from build123d import *

# Parameters (mm, degrees)
BOX006_W               = 2
BOX006_H               = 10
BOX006_DEPTH           = 30
BOX005_W               = 2
BOX005_H               = 10
BOX005_DEPTH           = 30
CYLINDER001_R          = 7.7
CYLINDER001_DEPTH      = 25
CYLINDER_R             = 7.7
CYLINDER_DEPTH         = 25
BOX004_W               = 32
BOX004_H               = 10
BOX004_DEPTH           = 15
BOX004_PLACEMENT_ANGLE = -37
BOX_W                  = 60
BOX_H                  = 10
BOX_DEPTH              = 15
CYLINDER002_R          = 11
CYLINDER002_DEPTH      = 25
CYLINDER003_R          = 11
CYLINDER003_DEPTH      = 25
BOX003_W               = 34
BOX003_H               = 10
BOX003_DEPTH           = 15
BOX003_PLACEMENT_ANGLE = 37
BOX002_W               = 34
BOX002_H               = 10
BOX002_DEPTH           = 15
BOX002_PLACEMENT_ANGLE = 37
CYLINDER005_R          = 7.2
CYLINDER005_DEPTH      = 40
CYLINDER004_R          = 7.2
CYLINDER004_DEPTH      = 40
BOX001_W               = 60
BOX001_H               = 10
BOX001_DEPTH           = 15
CHAMFER_SIZE           = 3


with BuildPart() as cube006:
    # Box006 → Box006 (new body)
    with BuildSketch(Plane(origin=(59, -15, 0), x_dir=(1, 0, 0), z_dir=(0, 0, 1))):
        with Locations((1, 5)):
            Rectangle(BOX006_W, BOX006_H)
    extrude(amount=BOX006_DEPTH)


with BuildPart() as cube005:
    # Box005 → Box005 (new body)
    with BuildSketch(Plane(origin=(-1, -15, 0), x_dir=(1, 0, 0), z_dir=(0, 0, 1))):
        with Locations((1, 5)):
            Rectangle(BOX005_W, BOX005_H)
    extrude(amount=BOX005_DEPTH)


with BuildPart() as cylinder001:
    # Cylinder001 → Cylinder001 (new body)
    with BuildSketch(Plane(origin=(60, 0, 0), x_dir=(1, 0, 0), z_dir=(0, 0, 1))):
        Circle(CYLINDER001_R)
    extrude(amount=CYLINDER001_DEPTH)


with BuildPart() as cylinder:
    # Cylinder → Cylinder (new body)
    with BuildSketch(Plane.XY):
        Circle(CYLINDER_R)
    extrude(amount=CYLINDER_DEPTH)


with BuildPart() as cube004:
    # Box004 → Box004 (new body)
    with BuildSketch(Plane.XY):
        with Locations((16, 5)):
            Rectangle(BOX004_W, BOX004_H)
    extrude(amount=BOX004_DEPTH)


with BuildPart() as cube004_1:
    # Box004 placement: moved
    add(cube004.part.moved(Location((23, 20, 0))).rotate(Axis((23, 20, 0), (0, 0, 1)), BOX004_PLACEMENT_ANGLE))


with BuildPart() as cube:
    # Box → Box (new body)
    with BuildSketch(Plane.XY):
        with Locations((30, 5)):
            Rectangle(BOX_W, BOX_H)
    extrude(amount=BOX_DEPTH)


with BuildPart() as cylinder002:
    # Cylinder002 → Cylinder002 (new body)
    with BuildSketch(Plane.XY):
        Circle(CYLINDER002_R)
    extrude(amount=CYLINDER002_DEPTH)


with BuildPart() as fusion003:
    # Cylinder003 → Cylinder003 (new body)
    with BuildSketch(Plane(origin=(60, 0, 0), x_dir=(1, 0, 0), z_dir=(0, 0, 1))):
        Circle(CYLINDER003_R)
    extrude(amount=CYLINDER003_DEPTH)

    # Fusion: union Cube, Cylinder002
    add(cube.part)
    add(cylinder002.part)

    # Fusion003: union Cube004
    add(cube004_1.part)


with BuildPart() as fusion004:
    # Box003 → Box003 (new body)
    with BuildSketch(Plane.XY):
        with Locations((17, 5)):
            Rectangle(BOX003_W, BOX003_H)
    extrude(amount=BOX003_DEPTH)


with BuildPart() as fusion004_1:
    # Box003 placement: moved
    add(fusion004.part.moved(Location((60, 0, 0))).rotate(Axis((60, 0, 0), (0, 0, 1)), BOX003_PLACEMENT_ANGLE))

    # Fusion004: union Fusion003
    add(fusion003.part)


with BuildPart() as cut003:
    # Box002 → Box002 (new body)
    with BuildSketch(Plane.XY):
        with Locations((17, 5)):
            Rectangle(BOX002_W, BOX002_H)
    extrude(amount=BOX002_DEPTH)


with BuildPart() as cut003_1:
    # Box002 placement: moved
    add(cut003.part.rotate(Axis((0, 0, 0), (0, 0, 1)), BOX002_PLACEMENT_ANGLE))

    # Fusion005: union Fusion004
    add(fusion004_1.part)

    # Cut: cut Cylinder
    add(cylinder.part, mode=Mode.SUBTRACT)

    # Cut001: cut Cylinder001
    add(cylinder001.part, mode=Mode.SUBTRACT)

    # Cut002: cut Cube005
    add(cube005.part, mode=Mode.SUBTRACT)

    # Cut003: cut Cube006
    add(cube006.part, mode=Mode.SUBTRACT)


with BuildPart() as cylinder005:
    # Cylinder005 → Cylinder005 (new body)
    with BuildSketch(Plane(origin=(60, 0, 0), x_dir=(1, 0, 0), z_dir=(0, 0, 1))):
        Circle(CYLINDER005_R)
    extrude(amount=CYLINDER005_DEPTH)


with BuildPart() as fusion001:
    # Cylinder004 → Cylinder004 (new body)
    with BuildSketch(Plane.XY):
        Circle(CYLINDER004_R)
    extrude(amount=CYLINDER004_DEPTH)

    # Fusion001: union Cylinder005
    add(cylinder005.part)


with BuildPart() as fusion006:
    # Box001 → Box001 (new body)
    with BuildSketch(Plane(origin=(0, -5, 0), x_dir=(1, 0, 0), z_dir=(0, 0, 1))):
        with Locations((30, 5)):
            Rectangle(BOX001_W, BOX001_H)
    extrude(amount=BOX001_DEPTH)

    # Fusion002: union Fusion001
    add(fusion001.part)

    # Chamfer
    chamfer_edges = [fusion006.edges().sort_by_distance(p)[0] for p in [
        (-7.2, 0, 40),
        (52.8, 0, 40),
    ]]
    chamfer(chamfer_edges, length=CHAMFER_SIZE)


with BuildPart() as fusion006_1:
    # Chamfer placement: moved
    add(fusion006.part.moved(Location((24, 25, 0))))

    # Fusion006: union Cut003
    add(cut003_1.part)


solid = fusion006_1.part
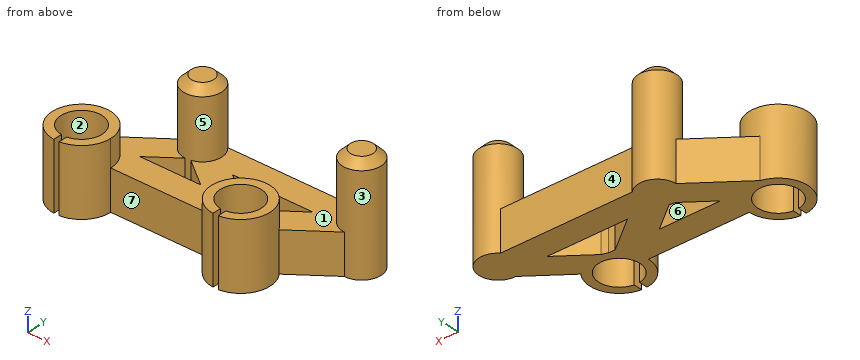
Model file for the job. Use its own axes, mm. Face numbers are marked on the shaded views. A direction names the side the tool comes from. Give positions to 0.01 mm unless a question says otherwise; leave off trailing zeros. Write each loop counter-clockwise with the first axis right and the second up, starting at its lowest first coordinate (ties: lowest second). Pieces come first, ordered by that corner, then holes. Notation, with made-up numbers: (-27, 15.5) -> (12, 15.5) arc R17 ccw to (12, 25.5) -> close; hole circle Ø5 at (-38.75, 52). An arc over 180 degrees is marked (long way). Write item = value, one per line.
(1) Probe line 1 along X through (y, z) = (0, 19); line 2 along X through (y, z) = (-3, 6); line 3 along Z through (x, y) = (36, 0.5). List the from-to ranges inside material, lowest first.
Determined:
line_1 = -11 to -7.7, 7.7 to 11, 49 to 52.3, 67.7 to 71
line_2 = -10.58 to -7.09, 7.09 to 10.58, 49.42 to 52.91, 67.09 to 70.58
line_3 = 0 to 15
(2) Slice it at D-D, the plane z = 5.5. Give the cut face in (x, y) (1 decimal), then the cut area to 3 significant figures.
Determined:
outline = (-2.4, 10.7) arc R11 ccw to (-1, -11) -> (-1, -7.6) arc R7.7 cw (long way) to (1, -7.6) -> (1, -11) arc R11 ccw to (11, 0) -> (49, 0) arc R11 ccw to (59, -11) -> (59, -7.6) arc R7.7 cw (long way) to (61, -7.6) -> (61, -11) arc R11 ccw to (68.8, 6.6) -> (83.6, 17.8) arc R7.2 ccw (long way) to (78.8, 30) -> (29.2, 30) arc R7.2 ccw to (16.8, 25.2) -> close; hole (13.3, 10) -> (36.3, 10) -> (25.7, 18) arc R7.2 cw to (23.6, 17.8) -> close; hole (39.6, 20) -> (52.9, 10) -> (55.4, 10) arc R11 cw to (57.6, 10.7) -> (69.9, 20) -> close
area = 2,080 mm2
(3) Mould opens along Y. For the marked faces 1, 2, 3 and 4 say: released by +Y, released by -Y, zero draft, split by the parting line, or undercut.
Determined:
face_1 = zero draft
face_2 = undercut
face_3 = split by the parting line
face_4 = released by +Y
(4) Flat gauge pins, fed straight in: P1, Ø10, axis at y = 17.5, z = 35.5, coming from the -X side; P2, Ø2, axis at x = 15, z = 12.5, coming from the -Y side; P3, Ø12, axis at x = 54, z = 5.5, coming from the -Y side. Where does each tip first touch, or does it go through?
Determined:
P1 = 17.25
P2 = 0
P3 = -10.95
(5) Slice it at A-A, the plane z = 16.5. Give the cut face in (x, y), then the cut area to 3 significant figures.
Determined:
outline = (-1, -10.95) -> (-1, -7.63) arc R7.7 cw (long way) to (1, -7.63) -> (1, -10.95) arc R11 ccw (long way) to start; circle Ø14.4 at (24, 25); (59, -10.95) -> (59, -7.63) arc R7.7 cw (long way) to (61, -7.63) -> (61, -10.95) arc R11 ccw (long way) to start; circle Ø14.4 at (84, 25)
area = 700 mm2
(6) Tool access for the marked faces 5, 6 and 7: list every direction of +Z, -Z, +X, -X, +Y, -Y with a clear straight run to the whole face (end or side of a thin tool).
Determined:
face_5 = +Z
face_6 = +Z, -Z
face_7 = +Z, -Z, -Y
(7) Slice it at B-B, the plane x = 4.5. Give the cut face in (y, z), then the cut area to 3 significant figures.
Determined:
outline = (-10.04, 0) -> (-6.25, 0) -> (-6.25, 25) -> (-10.04, 25) -> close; (6.25, 0) -> (15.91, 0) -> (15.91, 15) -> (10.04, 15) -> (10.04, 25) -> (6.25, 25) -> close
area = 278 mm2
(8) Slice it at C-C, the plane y = -1. Give the cut face in (x, z), then the cut area to 3 significant figures.
Determined:
outline = (-10.95, 0) -> (-7.63, 0) -> (-7.63, 25) -> (-10.95, 25) -> close; (7.63, 0) -> (10.95, 0) -> (10.95, 25) -> (7.63, 25) -> close; (49.05, 0) -> (52.37, 0) -> (52.37, 25) -> (49.05, 25) -> close; (67.63, 0) -> (70.95, 0) -> (70.95, 25) -> (67.63, 25) -> close
area = 332 mm2
